Study the drawing (mm; zero at the part's minimum x, y, z) and answer. Round coordinates to 2 decimals unless told otherwise and drop trailing zeros. Write each loop counter-clockwise with the first axis right and the second up, starting at its lowest first coordinate (ties: lowest second). Pieces come first, ordered by that corner, then holes.
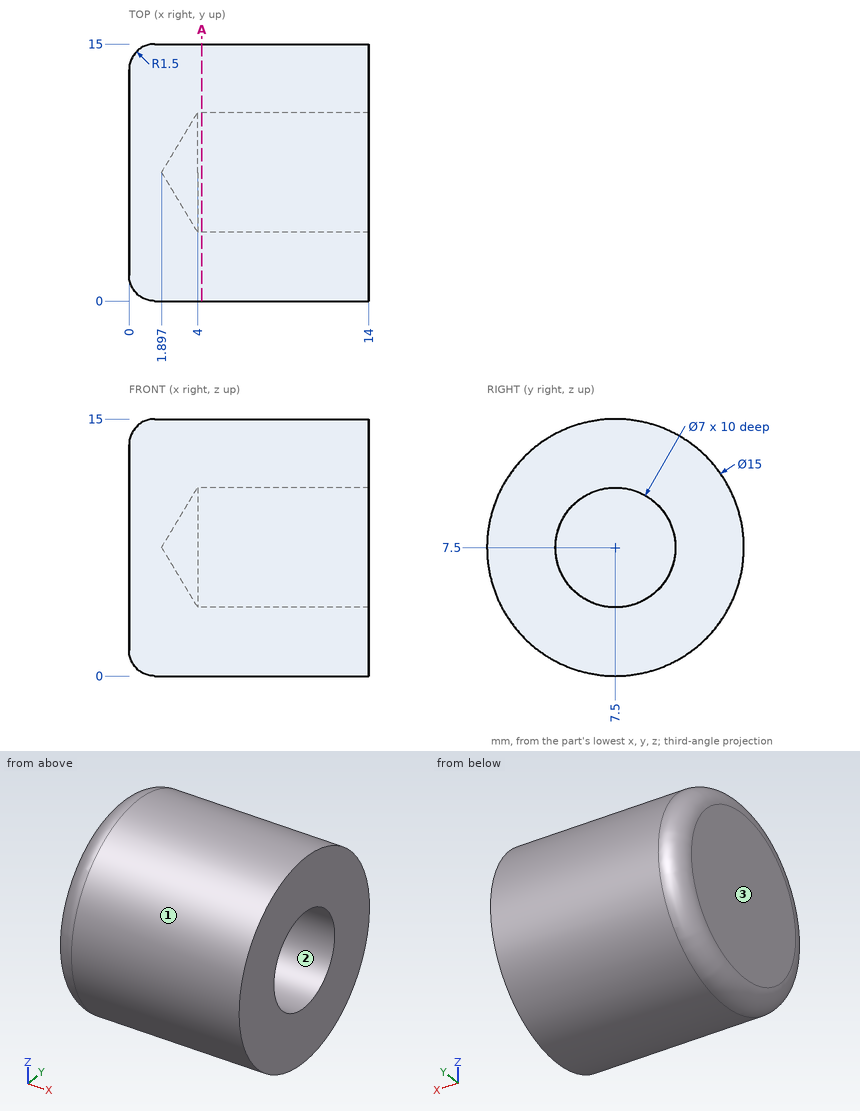
Q1. Given pin 1 (3 mm diameter, centred on x = 8.5, z = 9.5, fed in from +Y); pin 2 (2 mm diameter, centred on x = 7.5, z = 9, fed in from -Y); pin 3 (8 mm diameter, centred on x = 6, y = 13, fed in from -Z); pin 4 (8 mm diameter, centred on y = 7.5, z = 7.5, fed in from +X), each flat-ended and moving along its own axis, determine where each tip first touches the part or whether it passes through.
Q2. The mould has two halves that part along Z. Classify the marked faces 1, 2 and 3: +Z half, -Z half, draft (parallel to the pull), parting line (faces both ways), or undercut.
Q3. Find the intervals of material crossed by L1, parallel to Y at x = 8.5, z = 7.5; L2, parallel to Z at x = 10.25, y = 3, in increasing order.
Q4. Find section A-A (x = 4.25). Determine the outline of the cut face in (y, z), plus the area to 3 significant figures.
Report:
1. pin 1: stops at y = 14.98
1. pin 2: stops at y = 0.02
1. pin 3: stops at z = 0.15
1. pin 4: stops at x = 14
2. face 1: parting line
2. face 2: undercut
2. face 3: draft
3. L1: y = 0 to 4, 11 to 15
3. L2: z = 1.5 to 13.5
4. outline: circle Ø15 at (7.5, 7.5); hole circle Ø7 at (7.5, 7.5)
4. area: 138 mm2
